Geometry check sheet. Reference: the model listing, model coordinates, mm. Round coordinates to 2 decimals unless told otherwise and drop trailing zeros. Loops run counter-clockwise (first coordinate to the right, second up) from the corner with the lowest first, then second, coordinate; pieces in that order, holes last. Notation, with made-up numbers: (14.25, 57) - (40.25, 57) arc R26 cw to (40.25, 96) - close; hole circle Ø5 at (40.25, 29.25). An arc over 180 degrees is marked (long way). Write item = value, one per line.
```python
from build123d import *

# Parameters (mm, degrees)
F0_R     = 175
F0_R_2   = 140
F1_DEPTH = 37
F3_DEPTH = 64
F4_DEPTH = 40


with BuildPart() as f1:
    # F0 (on Front) → F1 (new body)
    with BuildSketch(Plane.XZ):
        Circle(F0_R)
        Circle(F0_R_2, mode=Mode.SUBTRACT)
    extrude(amount=F1_DEPTH)

    # F2 (on face) → F3 (cut)
    with BuildSketch(Plane.XZ.offset(37)):
        with BuildLine():
            Line((-134.6558720136, 127.5854463967), (-127.2283504649, 120.158007798))
            ThreePointArc((-127.2283504649, 120.158007798), (-123.7436867076, 123.7436867076), (-120.158007798, 127.2283504649))
            Line((-120.158007798, 127.2283504649), (-127.5854463967, 134.6558720136))
            ThreePointArc((-127.5854463967, 134.6558720136), (-134.703841816, 134.703841816), (-134.6558720136, 127.5854463967))
        make_face()
        with BuildLine():
            ThreePointArc((-123.3376217614, 116.267322546), (-119.8177388722, 114.8547352829), (-116.3190655052, 116.3190655052))
            ThreePointArc((-116.3190655052, 116.3190655052), (-114.8547352829, 119.8177388722), (-116.267322546, 123.3376217614))
            Line((-116.267322546, 123.3376217614), (-120.158007798, 127.2283504649))
            ThreePointArc((-120.158007798, 127.2283504649), (-123.7436867076, 123.7436867076), (-127.2283504649, 120.158007798))
            Line((-127.2283504649, 120.158007798), (-123.3376217614, 116.267322546))
        make_face()
        with BuildLine():
            ThreePointArc((-89.2769447092, 144.6683901164), (-86.2483562751, 142.021093318), (-82.25, 142.4611789225))
            ThreePointArc((-82.25, 142.4611789225), (-79.8696965491, 145.7038142279), (-80.6480286108, 149.6502971486))
            Line((-80.6480286108, 149.6502971486), (-83.1500538847, 153.9839879305))
            ThreePointArc((-83.1500538847, 153.9839879305), (-87.5003449373, 151.5542465121), (-91.7796966371, 149.0016351762))
            Line((-91.7796966372, 149.0016351762), (-89.397566175, 144.8749948502))
            Line((-89.397566175, 144.8749948502), (-89.2769447092, 144.6683901164))
        make_face()
    extrude(amount=-F3_DEPTH, mode=Mode.SUBTRACT)

    # F2 (on face) → F4 (cut)
    with BuildSketch(Plane.XZ.offset(37)):
        with BuildLine():
            ThreePointArc((0.5, 175), (-0.3535533906, 175.3535533906), (0, 174.5))
            ThreePointArc((0, 174.5), (0.3535533906, 174.6464466094), (0.5, 175))
        make_face()
        with BuildLine():
            ThreePointArc((-123.3376217614, 116.267322546), (-119.8177388722, 114.8547352829), (-116.3190655052, 116.3190655052))
            ThreePointArc((-116.3190655052, 116.3190655052), (-114.8547352829, 119.8177388722), (-116.267322546, 123.3376217614))
            Line((-116.267322546, 123.3376217614), (-127.5854463967, 134.6558720136))
            ThreePointArc((-127.5854463967, 134.6558720136), (-134.703841816, 134.703841816), (-134.6558720136, 127.5854463967))
            Line((-134.6558720136, 127.5854463967), (-123.3376217614, 116.267322546))
        make_face()
    extrude(amount=-F4_DEPTH, mode=Mode.SUBTRACT)


solid = f1.part
```
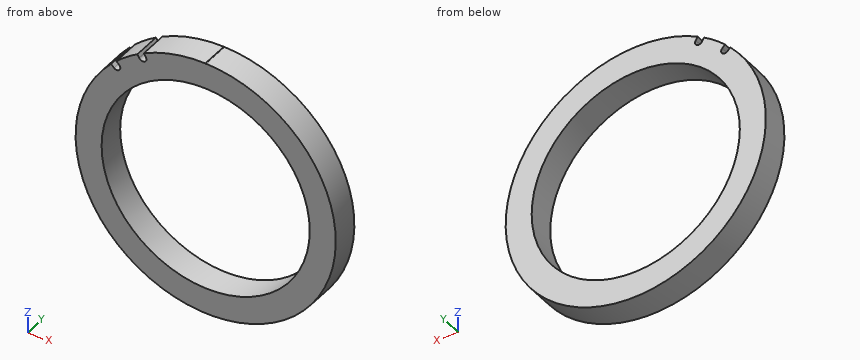
(1) Scan lines: L1, parallel to Z at x = 0, y = -21; L2, parallel to Z at x = -96, y = -23.5; L3, parallel to X at y = -16.5, z = -53. Record each from-to range of solid material in increasing order. Write a range as [from, to].
Answers follow:
L1 = [-175, -140], [140, 174.5]
L2 = [-146.32, -101.9], [101.9, 146.32]
L3 = [-166.78, -129.58], [129.58, 166.78]
(2) Section check B-B (z = 0). Enter the section's corners in (x, y).
Answers follow:
outline = (-175, -37) - (-140, -37) - (-140, 0) - (-175, 0) - close; (140, -37) - (175, -37) - (175, 0) - (140, 0) - close
(3) Section check A-A (y = -17). Enter the section's corners in (x, z) (3 decimals), then the cut area to 3 significant figures.
Answers follow:
outline = (-127.228, 120.158) arc R175 ccw (long way) to (0.5, 174.999) arc R0.5 cw to (-0.5, 174.999) arc R175 ccw to (-83.15, 153.984) - (-80.648, 149.65) arc R5 cw (long way) to (-89.277, 144.668) - (-89.398, 144.875) - (-91.78, 149.002) arc R175 ccw to (-120.158, 127.228) - (-116.267, 123.338) arc R5 cw to (-123.338, 116.267) - close; hole circle Ø280 at (0, 0)
area = 34,400 mm²
(4) Gauge pin test, flat ends, axial feed: pin 1 (10 mm diameter, centred on x = -86.5, y = -9.5, fed in from +Z); pin 2 (5 mm diameter, centred on y = -23, z = 31, fed in from +X); pin 3 (3 mm diameter, centred on x = -127.5, y = -8.5, fed in from -Z). Record the tip position at first contact, or that the pin passes through.
Answers follow:
pin_1 = 154.86
pin_2 = 172.66
pin_3 = -121.45
(5) Section check C-C (x = -54). Enter the section's corners in (y, z), then the cut area to 3 significant figures.
Answers follow:
outline = (-37, -166.46) - (0, -166.46) - (0, -129.17) - (-37, -129.17) - close; (-37, 129.17) - (0, 129.17) - (0, 166.46) - (-37, 166.46) - close
area = 2,760 mm²
